Could you check a few things on this model? Use its own coordinates, in mm. Round coordinates to 2 decimals unless told otherwise and drop trailing zeros. Order: outer loops, then holes, each group sorted by start corner. A loop starts at its lowest first (then second) coordinate and runs counter-clockwise, first axis right, second up. Notation, with made-up numbers: (37, 48.5) - (91, 48.5) arc R23 ccw to (91, 57.5) - close; hole circle Ø3 at (-25, 47.25). An arc over 180 degrees is marked (long way). Use one line per item in the form item = value.
from build123d import *

# Parameters (mm, degrees)
SKETCH_2_R          = 2.25
EXTRUDE_2_DEPTH     = 5
SKETCH_5_R          = 1.75
CUT_EXTRUDE_3_DEPTH = 213.190951739
SKETCH_8_R          = 1.75
CUT_EXTRUDE_5_DEPTH = 213.190951739


with BuildPart() as part:
    # 草圖2 → 填料-伸長2 (new body)
    with BuildSketch(Plane(origin=(0, 0, 0), x_dir=(1, 0, 0), z_dir=(0, 1, 0))):
        Polygon((-150, 150), (150, 150), (150, -50), (70, -150), (-70, -150), (-150, -50), align=None)
        with Locations(Location((-105, 121, 0), (0, 0, 270))):
            Circle(SKETCH_2_R, mode=Mode.SUBTRACT)
        with Locations(Location((-105, 79, 0), (0, 0, 270))):
            Circle(SKETCH_2_R, mode=Mode.SUBTRACT)
        with Locations(Location((-55, 79, 0), (0, 0, 270))):
            Circle(SKETCH_2_R, mode=Mode.SUBTRACT)
        with Locations(Location((-55, 121, 0), (0, 0, 270))):
            Circle(SKETCH_2_R, mode=Mode.SUBTRACT)
        with Locations(Location((55, 121, 0), (0, 0, 270))):
            Circle(SKETCH_2_R, mode=Mode.SUBTRACT)
        with Locations(Location((55, 79, 0), (0, 0, 270))):
            Circle(SKETCH_2_R, mode=Mode.SUBTRACT)
        with Locations(Location((105, 121, 0), (0, 0, 270))):
            Circle(SKETCH_2_R, mode=Mode.SUBTRACT)
        with Locations(Location((105, 79, 0), (0, 0, 270))):
            Circle(SKETCH_2_R, mode=Mode.SUBTRACT)
    extrude(amount=EXTRUDE_2_DEPTH)

    # 草圖5 → 除料-伸長3 (cut, through all)
    with BuildSketch(Plane(origin=(0, 5, 0), x_dir=(1, 0, 0), z_dir=(0, 1, 0))):
        with Locations(Location((0, 62, 0), (0, 0, 270))):
            Circle(SKETCH_5_R)
        with Locations(Location((-80, 62, 0), (0, 0, 270))):
            Circle(SKETCH_5_R)
        with Locations(Location((80, 62, 0), (0, 0, 90))):
            Circle(SKETCH_5_R)
        with Locations(Location((80, 138, 0), (0, 0, 270))):
            Circle(SKETCH_5_R)
        with Locations(Location((-80, 138, 0), (0, 0, 90))):
            Circle(SKETCH_5_R)
        with Locations(Location((0, 138, 0), (0, 0, 90))):
            Circle(SKETCH_5_R)
    extrude(amount=-CUT_EXTRUDE_3_DEPTH, mode=Mode.SUBTRACT)

    # 草圖8 → 除料-伸長5 (cut, through all)
    with BuildSketch(Plane(origin=(0, 5, 0), x_dir=(1, 0, 0), z_dir=(0, 1, 0))):
        with Locations(Location((-80, 121, 0), (0, 0, 270))):
            Circle(SKETCH_8_R)
        with Locations(Location((80, 121, 0), (0, 0, 90))):
            Circle(SKETCH_8_R)
        with Locations(Location((-135, -50, 0), (0, 0, 270))):
            Circle(SKETCH_8_R)
        with Locations(Location((-66.283544769, -135.895569039, 0), (0, 0, 270))):
            Circle(SKETCH_8_R)
        with Locations(Location((135, -50, 0), (0, 0, 90))):
            Circle(SKETCH_8_R)
        with Locations(Location((66.283544769, -135.895569039, 0), (0, 0, 90))):
            Circle(SKETCH_8_R)
    extrude(amount=-CUT_EXTRUDE_5_DEPTH, mode=Mode.SUBTRACT)


solid = part.part
Item 1: Will these pins go through, and if not, where does the flat tip stop? P1, Ø7, axis at x = -105, z = -121, coming from the -Y side; P2, Ø3, axis at x = -72, y = 2, coming from the +Z side (3 decimals).
Found:
P1 = 0
P2 = 149.375
Item 2: Imagine slicing it at B-B on x = -116. Please give me the cut outline in (y, z).
Found:
outline = (0, -150) - (5, -150) - (5, 92.5) - (0, 92.5) - close
Item 3: Imagine slicing it at A-A on y = 3.45. State how many separate pieces and enclosed holes the cut face has, plus the area to 3 significant figures.
Found:
separate_pieces = 1
enclosed_holes = 20
area = 81,800 mm2
Item 4: Imagine slicing it at C-C on z = 109. Please give me the cut outline in (x, y), plus the area to 3 significant figures.
Found:
outline = (-102.8, 0) - (102.8, 0) - (102.8, 5) - (-102.8, 5) - close
area = 1,030 mm2
Item 5: I need wall thicknesses on L1, parallel to X at y = 4, z = -136.5; L2, parallel to Z at x = 80, y = 3.5; L3, parallel to Z at x = -105.5, y = 2.75 (3 decimals). Which ranges of each line are inside material? Lowest first, please.
Found:
L1 = -150 to -80.9, -79.1 to -0.9, 0.9 to 79.1, 80.9 to 150
L2 = -150 to -139.75, -136.25 to -122.75, -119.25 to -63.75, -60.25 to 137.5
L3 = -150 to -123.194, -118.806 to -81.194, -76.806 to 105.625
